Solid Edge part; units mm, degrees
sketch "Sketch1" plane through (0, 0, 0) normal (0, 0, 1) x (1, 0, 0)
  line L0 (-42.5, -42.75) -> (42.5, -42.75)
  line L1 (42.5, -42.75) -> (42.5, 42.75)
  line L2 (42.5, 42.75) -> (-42.5, 42.75)
  line L3 (-42.5, 42.75) -> (-42.5, -42.75)
extrude "Protrusion1" add sketch "Sketch1" against normal blind 25
sketch "Sketch2" plane through (42.5, 0, -12.5) normal (1, 0, 0) x (0, 1, 0)
  line L0 (-42.75, 12.5) -> (-23.1, 12.5)
  arc A0 (-23.1, 12.5) -> (-42.75, -8.5) centre (-78.4621, 44.6097) cw
  line L1 (-42.75, 12.5) -> (-42.75, -8.5)
extrude "ExtrudedCutout_2" cut sketch "Sketch2" against normal blind 85
fillet "Round_1" radius 2 1 edges at (0, -42.75, -21)
sketch "Sketch3" plane through (42.5, 0, -12.5) normal (1, 0, 0) x (0, 1, 0)
  line L0 (42.75, 12.5) -> (23.1, 12.5)
  arc A0 (23.1, 12.5) -> (42.75, -8.5) centre (78.4621, 44.6097) ccw
  line L1 (42.75, 12.5) -> (42.75, -8.5)
extrude "ExtrudedCutout_3" cut sketch "Sketch3" against normal blind 85
fillet "Round_2" radius 2 1 edges at (0, 42.75, -21)
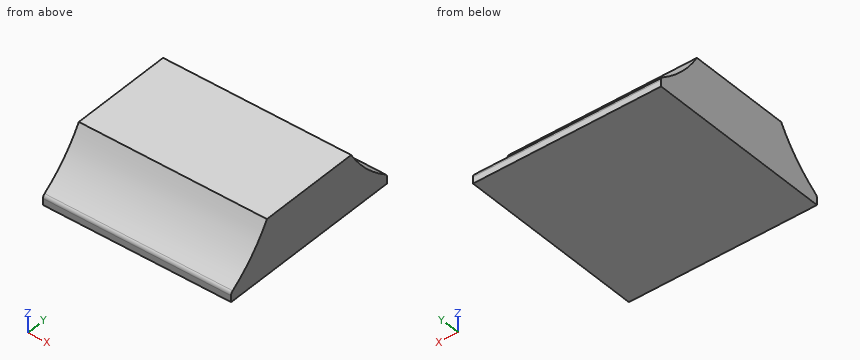
Here's how the part is built. I have some questions about the finished solid (model axes, mm). Coordinates: 2 decimals unless noted, no trailing zeros. Write each loop counter-clockwise with the first axis right and the second up, starting at its lowest first coordinate (ties: lowest second). Pieces come first, ordered by that corner, then holes.
Item 1: If I drill on line 1 (Y direction, x = -35, z = -4.25); line 2 (Y direction, x = 18, z = -10); line 3 (Z direction, x = 0.5, y = 23.5), over which ranges is the centre line in solid material (lowest first)?
Item 2: I want a section at B-B on z = -13.25. Write out the boundary of the cut face in (x, y).
Item 3: I want a section at A-A on x = 3. Write out the boundary of the cut face in (y, z).
Item 4: I want a section at C-C on y = 35.5. Write out the boundary of the cut face in (x, z), and give its area (3 significant figures).
Item 5: Will these pins go through, and if not, where does the flat tip stop? pin 1 (4 mm diameter, centred on x = 20, z = -6, fed in from -Y); pin 2 (3 mm diameter, centred on x = 14, y = -30, fed in from +Z); pin 3 (1.5 mm diameter, centred on x = 12.5, z = -3.5, fed in from +Y).
Findings below:
1. line 1: y = -25.79 to 25.79
1. line 2: y = -30.27 to 30.27
1. line 3: z = -25 to -0.68
2. outline: (-42.5, -33.31) - (42.5, -33.31) - (42.5, 33.31) - (-42.5, 33.31) - close
3. outline: (-42.75, -25) - (42.75, -25) - (42.75, -22.05) arc R2 ccw to (41.89, -20.41) arc R64 cw to (23.1, 0) - (-23.1, 0) arc R64 cw to (-41.89, -20.41) arc R2 ccw to (-42.75, -22.05) - close
4. outline: (-42.5, -25) - (42.5, -25) - (42.5, -15.33) - (-42.5, -15.33) - close
4. area: 822 mm2
5. pin 1: stops at y = -28.59
5. pin 2: stops at z = -7.89
5. pin 3: stops at y = 25.79
